Can you work these out from the model? Positions are in its coordinate system, mm. A direction names the side the tool comes from. Give positions to 0.01 mm unless a question says otherwise; leave off trailing zeros. Order: outer loops, then holes, each group sorted by start corner. A loop starts at its lowest first (then second) coordinate and runs counter-clockwise, first axis right, second up. Notation, with made-up numbers: M 16,89.25 L 38,89.25 A21 cw 38,103.25 Z; hole C 69.25,33 d6. An arc over 180 degrees is marked long. Use one line per item in the form item = value. Start each with the question number.
1. I want a section at C-C, the plane y = 11. List the corners of the cut face in (x, z) for me.
2. I want a section at B-B, the plane x = 11. List the corners of the cut face in (y, z) for me, and give its area (3 significant figures).
3. I want a section at D-D, the plane x = 41.5. List the corners of the cut face in (y, z) for me, and give its area (3 significant figures).
4. Will these pins go through, and if not, where does the flat tip stop? P1, Ø2, axis at y = 0, z = -3, coming from the -X side; P2, Ø5, axis at x = 23, z = 4, coming from the +Y side; P3, Ø5, axis at x = 1.5, y = 8, coming from the +Z side.
5. I want a section at A-A, the plane z = 0. List the corners of the cut face in (x, y) for me.
6. I need wall thicknesses on L1, parallel to Y at x = 24.5, z = 3.5; L2, parallel to Y at x = 40, z = -5; L3, parallel to X at y = 12.5, z = -4.75. Which ranges of each line are inside material? Lowest first, please.
7. For faces 1 (the face through (0, 15, 0)), 2 (the face through (34.143, -4.93, -1.301)), 3 (the face through (1.802, 9.93, 5.723)), which set-ups out of +Z, -Z, +X, -X, +Y, -Y let a thin tool reach every point of the face, with its end or its side?
```python
from build123d import *

# Parameters (mm, degrees)
BOSS_EXTRUDE1_DEPTH = 5
SKETCH1_3_R         = 6
BOSS_EXTRUDE2_DEPTH = 15
SKETCH1_4_R         = 6
BOSS_EXTRUDE3_DEPTH = 10


with BuildPart() as part:
    # Sketch1 → Boss-Extrude1 (new body)
    with BuildSketch(Plane(origin=(0, 0, 0), x_dir=(1, 0, 0), z_dir=(0, 1, 0))):
        with BuildLine():
            Line((0, 8), (40, 8))
            ThreePointArc((40, 8), (48, 0), (40, -8))
            Line((40, -8), (0, -8))
            ThreePointArc((0, -8), (-8, 0), (0, 8))
        make_face()
    extrude(amount=BOSS_EXTRUDE1_DEPTH)

    # Sketch1_3 → Boss-Extrude2 (add)
    with BuildSketch(Plane(origin=(0, 0, 0), x_dir=(1, 0, 0), z_dir=(0, 1, 0))):
        with Locations(Location((0, 0, 0), (0, 0, 270))):
            Circle(SKETCH1_3_R)
    extrude(amount=BOSS_EXTRUDE2_DEPTH)

    # Sketch1_4 → Boss-Extrude3 (add)
    with BuildSketch(Plane(origin=(0, 0, 0), x_dir=(1, 0, 0), z_dir=(0, 1, 0))):
        with Locations(Location((40, 0, 0), (0, 0, 270))):
            Circle(SKETCH1_4_R)
    extrude(amount=-BOSS_EXTRUDE3_DEPTH)


solid = part.part
```
Check result:
q1.outline = C 0,0 d12
q2.outline = M 0,-8 L 5,-8 L 5,8 L 0,8 Z
q2.area = 80.0 mm2
q3.outline = M -10,-5.81 L 0,-5.81 L 0,-7.86 L 5,-7.86 L 5,7.86 L 0,7.86 L 0,5.81 L -10,5.81 Z
q3.area = 195 mm2
q4.P1 = -7.75
q4.P2 = 5
q4.P3 = 6
q5.outline = M -8,0 L 34,0 L 34,-10 L 46,-10 L 46,0 L 48,0 L 48,5 L 6,5 L 6,15 L -6,15 L -6,5 L -8,5 Z
q6.L1 = 0 to 5
q6.L2 = -10 to 5
q6.L3 = -3.67 to 3.67
q7.face_1 = +Z, -Z, +X, -X, +Y
q7.face_2 = -Y
q7.face_3 = +Y
